Answer from the drawing. Dimensions are ordinates in mm from the lowest x, y and z of the part. Coordinates: 2 decimals unless noted, no trailing zeros. Write each loop counter-clockwise with the first axis right and the second up, starting at its lowest first coordinate (ties: lowest second). Pieces come first, ordered by that corner, then holes. Notation, with made-up numbers: (82.25, 86.5) -> (120.25, 86.5) arc R21 ccw to (120.25, 112.5) -> close; hole circle Ø5 at (-17, 65). An arc over 180 degrees is marked (long way). Answer as a JSON object with one key per item and string values. Group by question number.
(1) Find section B-B (y = 82). Give the vertices of the cut face in (x, z).
(2) A flat-ended cylindrical pin translates along its axis: P1, Ø4, axis at x = 55, y = 82, coming from the -Z side. Find the tip coordinate at first contact, or state that the pin passes through.
(3) For a pull along Z with two mould halves and no side action, classify the marked faces 1, 2 and 3 as +Z half, -Z half, draft (parallel to the pull), parting line (faces both ways), or undercut.
(4) Find section A-A (x = 25). Give the vertices of the cut face in (y, z).
(5) Straight lines are drawn through the part: L1, parallel to Y at x = 25, z = 5; L2, parallel to X at y = 69, z = 5; L3, parallel to Y at x = 59, z = 4.75. For each, find the intervals that lie inside material, in ascending order.
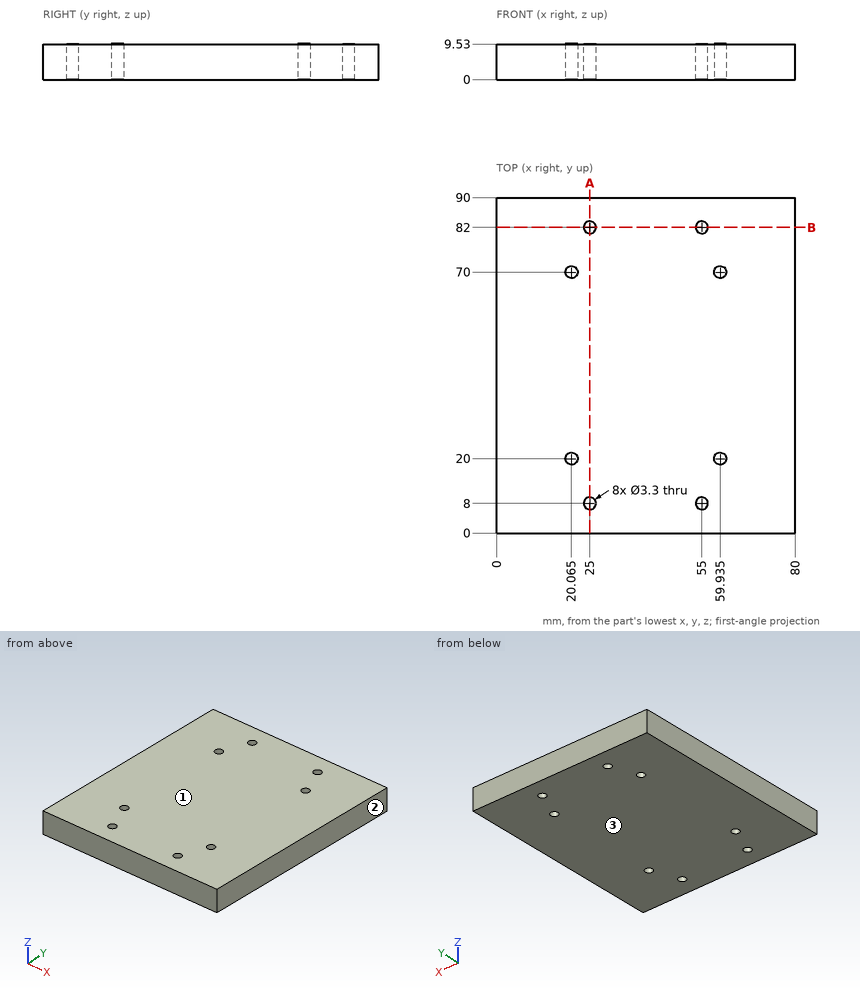
Results below:
{
 "1": {"outline": "(0, 0) -> (23.35, 0) -> (23.35, 9.53) -> (0, 9.53) -> close; (26.65, 0) -> (53.35, 0) -> (53.35, 9.53) -> (26.65, 9.53) -> close; (56.65, 0) -> (80, 0) -> (80, 9.53) -> (56.65, 9.53) -> close"},
 "2": {"P1": "stops at z = 0"},
 "3": {"face 1": "+Z half", "face 2": "draft", "face 3": "-Z half"},
 "4": {"outline": "(0, 0) -> (6.35, 0) -> (6.35, 9.53) -> (0, 9.53) -> close; (9.65, 0) -> (80.35, 0) -> (80.35, 9.53) -> (9.65, 9.53) -> close; (83.65, 0) -> (90, 0) -> (90, 9.53) -> (83.65, 9.53) -> close"},
 "5": {"L1": "y = 0 to 6.35, 9.65 to 80.35, 83.65 to 90", "L2": "x = 0 to 18.75, 21.38 to 58.62, 61.25 to 80", "L3": "y = 0 to 18.64, 21.36 to 68.64, 71.36 to 90"}
}
